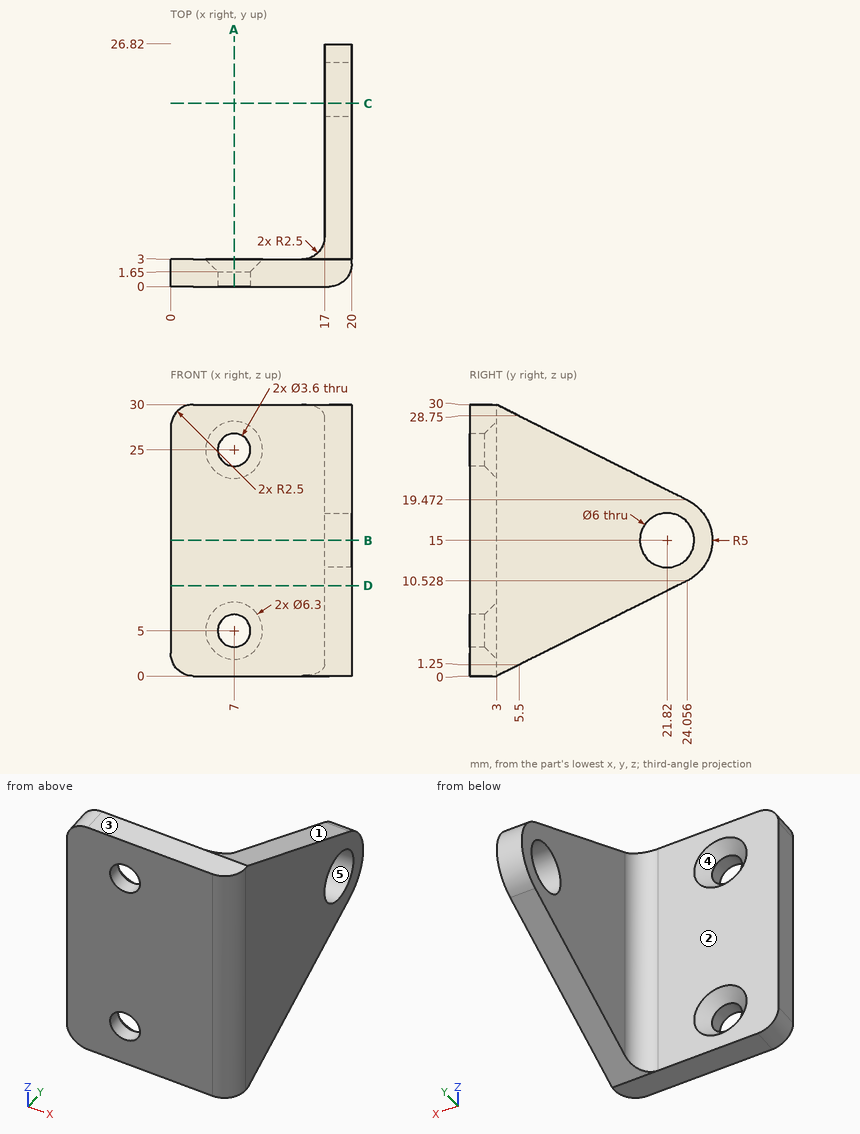
Verification items for this drawing (mm, ordinates from the low corner). A direction names the side the tool comes from. Coordinates: 2 decimals unless noted, no trailing zeros. Loops run counter-clockwise (first coordinate to the right, second up) from the corner with the lowest first, then second, coordinate; pieces in that order, holes last. Notation, with made-up numbers: (38, -3) -> (55, -3) arc R32 ccw to (55, 36) -> close; hole circle Ø1 at (58, -35). An arc over 180 degrees is marked (long way). Put each result on its own line as item: value.
1. Section check D-D, the plane z = 10. Record the boundary of the cut face in (x, y), then the cut area to 3 significant figures.
Result set:
outline: (0, 0) -> (17.5, 0) arc R2.5 ccw to (20, 2.5) -> (20, 23) -> (17, 23) -> (17, 5.5) arc R2.5 cw to (14.5, 3) -> (0, 3) -> close
area: 120 mm^2
2. Mould release check, pull along Y, two halves, no side actions. Record for the marked faces 3, 4 and 5: pulls with the +Y half, pulls with the -Y half, needs draft (parallel to the pull), parting line crosses it, or undercut.
Result set:
face 3: needs draft
face 4: pulls with the +Y half
face 5: undercut
3. Section check A-A, the plane x = 7. Record the boundary of the cut face in (y, z).
Result set:
outline: (0, 0) -> (3, 0) -> (3, 1.85) -> (1.65, 3.2) -> (0, 3.2) -> close; (0, 6.8) -> (1.65, 6.8) -> (3, 8.15) -> (3, 21.85) -> (1.65, 23.2) -> (0, 23.2) -> close; (0, 26.8) -> (1.65, 26.8) -> (3, 28.15) -> (3, 30) -> (0, 30) -> close
4. Tool access check on the marked faces 1 and 2. Record the directions out of +Z, -Z, +X, -X, +Y, -Y that give a thin tool (end or side, any length) a straight path to the whole face; none if there is none.
Result set:
face 1: +Z, +X, -X, +Y
face 2: +Z, -Z, -X, +Y
5. Section check B-B, the plane z = 15. Record the boundary of the cut face in (x, y).
Result set:
outline: (0, 0) -> (17.5, 0) arc R2.5 ccw to (20, 2.5) -> (20, 18.82) -> (17, 18.82) -> (17, 5.5) arc R2.5 cw to (14.5, 3) -> (0, 3) -> close; (17, 24.82) -> (20, 24.82) -> (20, 26.82) -> (17, 26.82) -> close
6. Section check C-C, the plane y = 20.25. Record the boundary of the cut face in (x, z) (1 decimal), then the cut area to 3 significant figures.
Result set:
outline: (17, 8.6) -> (20, 8.6) -> (20, 12.4) -> (17, 12.4) -> close; (17, 17.6) -> (20, 17.6) -> (20, 21.4) -> (17, 21.4) -> close
area: 22.9 mm^2
7. Thickness scan on line 1 (Z direction, x = 7, y = 0.6); line 2 (X direction, y = 9.5, z = 25.5); line 3 (Y direction, x = 11.5, z = 6.25). Record the ranges inside material, lowest first.
Result set:
line 1: z = 0 to 3.2, 6.8 to 23.2, 26.8 to 30
line 2: x = 17 to 20
line 3: y = 0 to 3
8. Gauge pin test, flat ends, axial feed: P1, Ø5, axis at x = 17.5, y = 18, coming from the +Z side; P2, Ø4.5, axis at x = 10.5, z = 20.5, coming from the +Y side; P3, Ø6.5, axis at y = 13.5, z = 17.5, coming from the -X side. Record the tip position at first contact, or that the pin passes through.
Result set:
P1: stops at z = 23.75
P2: stops at y = 3
P3: stops at x = 17
